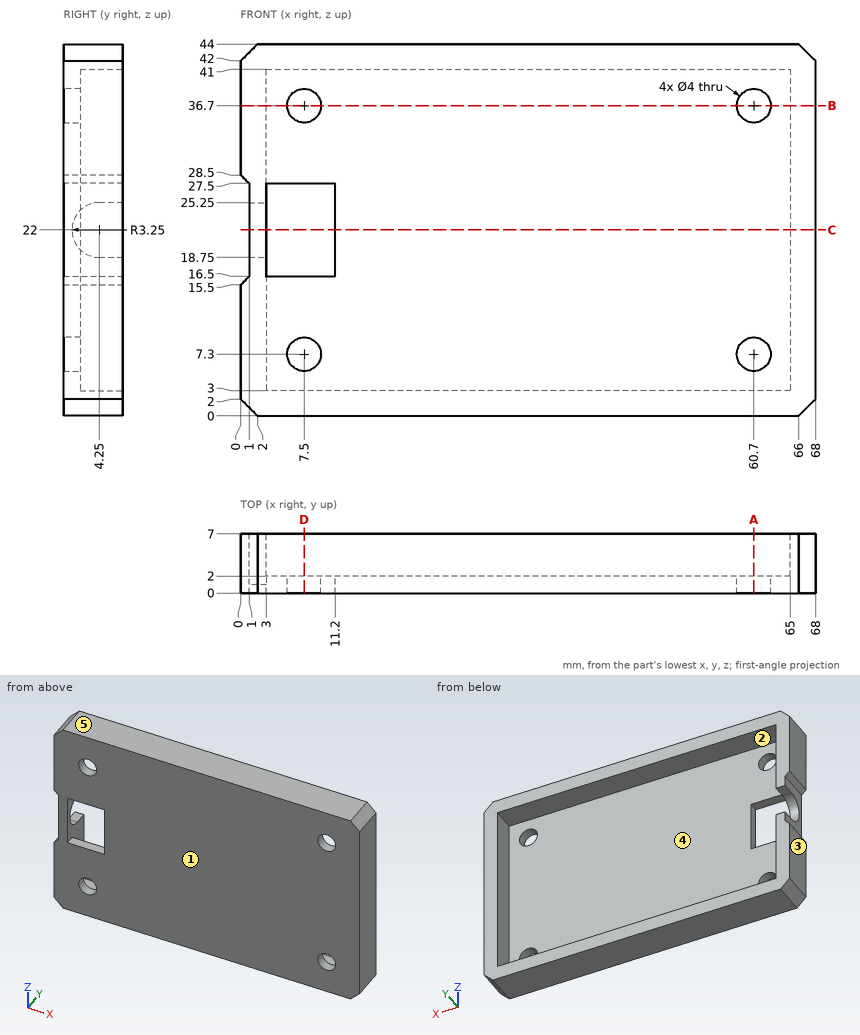
Could you check a few things on this drawing? It's one solid part, dimensions in mm from its lowest x, y, z. A direction names the side the tool comes from. Give positions to 0.01 mm unless a question says otherwise; leave off trailing zeros. Order: outer loops, then holes, each group sorted by start corner. A loop starts at its lowest first (then second) coordinate and runs counter-clockwise, first axis right, second up.
1. Suppose I cut it at A-A (x = 60.7). Write out the boundary of the cut face in (y, z).
Answers below:
outline: (0, 0) - (7, 0) - (7, 3) - (2, 3) - (2, 5.3) - (0, 5.3) - close; (0, 9.3) - (2, 9.3) - (2, 34.7) - (0, 34.7) - close; (0, 38.7) - (2, 38.7) - (2, 41) - (7, 41) - (7, 44) - (0, 44) - close
2. Suppose I cut it at B-B (z = 36.7). Write out the boundary of the cut face in (x, y).
Answers below:
outline: (0, 0) - (5.5, 0) - (5.5, 2) - (3, 2) - (3, 7) - (0, 7) - close; (9.5, 0) - (58.7, 0) - (58.7, 2) - (9.5, 2) - close; (62.7, 0) - (68, 0) - (68, 7) - (65, 7) - (65, 2) - (62.7, 2) - close
3. Which directions (+Z, -Z, +X, -X, +Y, -Y) give clear straight access to the entire face, cutting with the end or side of a thin tool? Please do the marked faces 4 and 5.
Answers below:
face 4: +Y
face 5: +Z, +X, -X, +Y, -Y
4. Suppose I cut it at D-D (x = 7.5). Write out the boundary of the cut face in (y, z).
Answers below:
outline: (0, 0) - (7, 0) - (7, 3) - (2, 3) - (2, 5.3) - (0, 5.3) - close; (0, 9.3) - (2, 9.3) - (2, 16.5) - (0, 16.5) - close; (0, 27.5) - (2, 27.5) - (2, 34.7) - (0, 34.7) - close; (0, 38.7) - (2, 38.7) - (2, 41) - (7, 41) - (7, 44) - (0, 44) - close
5. For pin 1 (2.5 mm diameter, centred on x = 60.7, z = 36.7, fed in from +Y); pin 2 (6.5 mm diameter, centred on x = 7.5, z = 7.3, fed in from +Y), each with a flat end and sliding along its axis, tell me the tip position at first contact or that it passes through.
Answers below:
pin 1: passes through
pin 2: stops at y = 2
6. I need wall thicknesses on L1, parallel to X at y = 1.05, z = 7.3; L2, parallel to Z at x = 60.7, y = 0.8; L3, parallel to X at y = 4, z = 5. Which ranges of each line are inside material? Lowest first, please.
Answers below:
L1: x = 0 to 5.5, 9.5 to 58.7, 62.7 to 68
L2: z = 0 to 5.3, 9.3 to 34.7, 38.7 to 44
L3: x = 0 to 3, 65 to 68
7. Suppose I cut it at C-C (z = 22). Write out the boundary of the cut face in (x, y), plus the area to 3 significant figures.
Answers below:
outline: (1, 0) - (3, 0) - (3, 1) - (1, 1) - close; (11.2, 0) - (68, 0) - (68, 7) - (65, 7) - (65, 2) - (11.2, 2) - close
area: 131 mm2
8. Thinking about a two-plate mould opening in X: for the marked faces 1, 2 and 3, which applies, +X half, -X half, draft (parallel to the pull), parting line (faces both ways), or undercut?
Answers below:
face 1: draft
face 2: undercut
face 3: -X half
